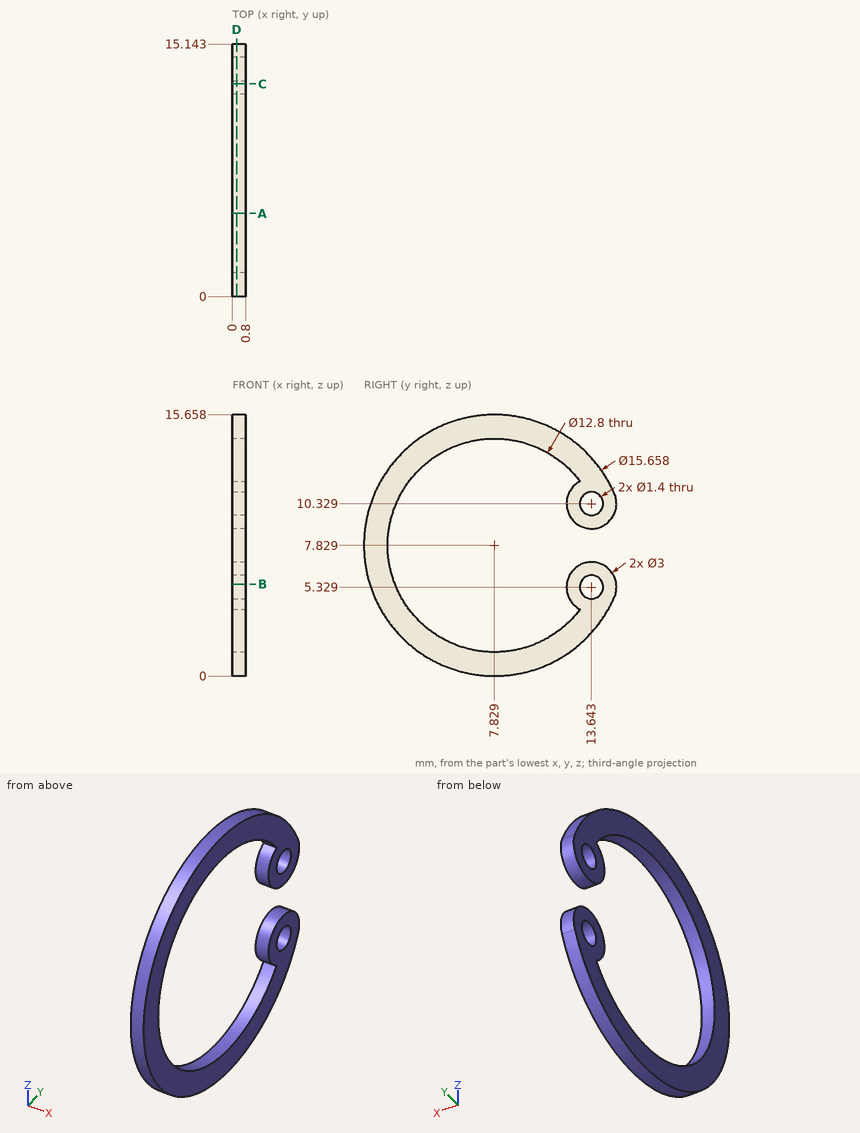
Print and shaded views of the part. All mm, measured from the part's lowest x, y and z. Round coordinates to 2 decimals unless told otherwise and drop trailing zeros. Write each loop counter-clockwise with the first axis right and the second up, starting at its lowest first coordinate (ties: lowest second). Pieces come first, ordered by that corner, then holes. Notation, with made-up numbers: (-10, 63) - (41, 63) arc R16 cw to (41, 82) - close; hole circle Ø4 at (38, 68). An arc over 180 degrees is marked (long way). One line per item, written item: value.
(1) Drop flat-ended pins along their axis: P1, Ø0.8, axis at y = 13.64, z = 10.33, coming from the -X side; P2, Ø8, axis at y = 6.5, z = 13.5, coming from the -X side. Give the stop position or say it passes through.
Values follow:
P1: passes through
P2: stops at x = 0
(2) Cut at B-B, the plane z = 5.5. Give the cut face in (x, y).
Values follow:
outline: (0, 0.35) - (0.8, 0.35) - (0.8, 1.87) - (0, 1.87) - close; (0, 12.15) - (0.8, 12.15) - (0.8, 12.96) - (0, 12.96) - close; (0, 14.32) - (0.8, 14.32) - (0.8, 15.13) - (0, 15.13) - close
(3) Cut at D-D, the plane x = 0.25. Give the cut face in (y, z).
Values follow:
outline: (12.95, 4) arc R6.4 cw (long way) to (12.95, 11.66) arc R1.5 ccw (long way) to (15.02, 10.92) arc R7.83 ccw (long way) to (15.02, 4.74) arc R1.5 ccw (long way) to start; hole circle Ø1.4 at (13.64, 5.33); hole circle Ø1.4 at (13.64, 10.33)
(4) Cut at A-A, the plane y = 5. Give the cut face in (x, z).
Values follow:
outline: (0, 0.53) - (0.8, 0.53) - (0.8, 2.09) - (0, 2.09) - close; (0, 13.57) - (0.8, 13.57) - (0.8, 15.13) - (0, 15.13) - close
(5) Wall check: probe 1 along Y at (x, z) = (0.1, 10.5) (1 decimal); probe 2 along Y at (x, z) = (0.7, 5) (1 decimal); probe 3 along Z at (x, y) = (0.15, 2.75) (1 decimal). Give the ranges that are in metal, low to high.
Values follow:
probe 1: y = 0.5 to 2, 12.2 to 13, 14.3 to 15.1
probe 2: y = 0.5 to 2.1, 12.2 to 13, 14.3 to 15.1
probe 3: z = 1.9 to 3.9, 11.7 to 13.8
(6) Cut at C-C, the plane y = 12.75. Give the cut face in (x, z).
Values follow:
outline: (0, 1.74) - (0.8, 1.74) - (0.8, 3.74) - (0, 3.74) - close; (0, 4.12) - (0.8, 4.12) - (0.8, 6.53) - (0, 6.53) - close; (0, 9.12) - (0.8, 9.12) - (0.8, 11.53) - (0, 11.53) - close; (0, 11.92) - (0.8, 11.92) - (0.8, 13.92) - (0, 13.92) - close
